```python
from build123d import *

# Parameters (mm, degrees)
SKETCH1_W           = 29
SKETCH1_H           = 45
SKETCH1_W_2         = 25
SKETCH1_H_2         = 41
BOSS_EXTRUDE1_DEPTH = 3
SKETCH2_W           = 29
SKETCH2_H           = 45
BOSS_EXTRUDE2_DEPTH = 1
SKETCH4_W           = 24.8
SKETCH4_H           = 2
BOSS_EXTRUDE3_DEPTH = 28


with BuildPart() as part:
    # Sketch1 → Boss-Extrude1 (new body)
    with BuildSketch(Plane(origin=(0, 0, 0), x_dir=(1, 0, 0), z_dir=(0, 1, 0))):
        Rectangle(SKETCH1_W, SKETCH1_H)
        Rectangle(SKETCH1_W_2, SKETCH1_H_2, mode=Mode.SUBTRACT)
    extrude(amount=BOSS_EXTRUDE1_DEPTH)

    # Sketch2 → Boss-Extrude2 (add)
    with BuildSketch(Plane(origin=(0, 3, 0), x_dir=(1, 0, 0), z_dir=(0, 1, 0))):
        Rectangle(SKETCH2_W, SKETCH2_H)
    extrude(amount=BOSS_EXTRUDE2_DEPTH)

    # Sketch4 → Boss-Extrude3 (add)
    with BuildSketch(Plane(origin=(0, 0, 0), x_dir=(-1, 0, 0), z_dir=(0, -1, 0))):
        with Locations((0.1, 21.5)):
            Rectangle(SKETCH4_W, SKETCH4_H)
    extrude(amount=BOSS_EXTRUDE3_DEPTH)


solid = part.part
```
Geometry: final body of the model. Coordinates: model frame, mm. A direction names the side the tool comes from. Coordinates: 2 decimals unless noted, no trailing zeros. Order: outer loops, then holes, each group sorted by start corner. A loop starts at its lowest first (then second) coordinate and runs counter-clockwise, first axis right, second up. Notation, with made-up numbers: (15.25, 31) - (58.25, 31) arc R22 cw to (58.25, 67) - close; hole circle Ø6 at (22.5, -23.5). An arc over 180 degrees is marked (long way). Write each question's results on one line, items separated by ' | '.
1) Section B-B, the plane z = -1.5. Return loops of the section in (x, y), plus the area to 3 significant figures.
Results list:
outline: (-14.5, 0) - (-12.5, 0) - (-12.5, 3) - (12.5, 3) - (12.5, 0) - (14.5, 0) - (14.5, 4) - (-14.5, 4) - close | area: 41.0 mm^2
2) Pin query (flat end, axial travel): pin 1 (6 mm diameter, centred on x = -11.5, y = -5.5, fed in from +Z); pin 2 (8.5 mm diameter, centred on x = -2, z = -2, fed in from -Y); pin 3 (1.6 mm diameter, centred on y = -10, z = -21, fed in from -X). Return the tip coordinate at first contact, or that it passes through.
Results list:
pin 1: z = -20.5 | pin 2: y = 3 | pin 3: x = -12.5
3) Section A-A, the plane x = 3. Return loops of the section in (y, z).
Results list:
outline: (-28, -22.5) - (4, -22.5) - (4, 22.5) - (0, 22.5) - (0, 20.5) - (3, 20.5) - (3, -20.5) - (-28, -20.5) - close
4) Line query: line 1 (Y direction, x = 2.25, z = 11); line 2 (Z direction, x = 4.75, y = -21); line 3 (Z direction, x = 5.75, y = 1.5). Output: solid intervals per line, ascending. Write a range as from..to.
Results list:
line 1: 3..4 | line 2: -22.5..-20.5 | line 3: -22.5..-20.5, 20.5..22.5
5) Section C-C, the plane y = -13. Return loops of the section in (x, z).
Results list:
outline: (-12.5, -22.5) - (12.3, -22.5) - (12.3, -20.5) - (-12.5, -20.5) - close
6) Pull-direction query (Z, two-part tool) for faces 4 (the flat face through (12.5, 1, 0)), 5 (the flat face through (0, -12, -22.5)), 6 (the flat face through (12.3, -14, -21)), 7 (the flat face through (0, 2, 22.5)); classes: pulls with the +Z half, pulls with the -Z half, needs draft (parallel to the pull), parting line crosses it, or undercut.
Results list:
face 4: undercut | face 5: pulls with the -Z half | face 6: needs draft | face 7: pulls with the +Z half
7) Set-up query: faces 1 (the flat face through (-14.5, 2, 0)), 2 (the flat face through (-12.5, -14, -21)), 3 (the flat face through (0, 1, 20.5)). Return all of +Z, -Z, +X, -X, +Y, -Y with unobstructed straight access to the full face (end or side cutting, diameter ignored); none if empty.
Results list:
face 1: +Z, -Z, -X, +Y, -Y | face 2: +Z, -Z, -X, -Y | face 3: -Y
